from build123d import *

# Parameters (mm, degrees)
SKETCH1_W           = 604.52
SKETCH1_H           = 251.46
BOSS_EXTRUDE1_DEPTH = 35.56
SKETCH2_W           = 601.98
SKETCH2_H           = 248.92
CUT_EXTRUDE1_DEPTH  = 34.29
SKETCH3_W           = 101.6
SKETCH3_H           = 6.35
BOSS_EXTRUDE2_DEPTH = 30.48
SKETCH4_W           = 88.9
SKETCH4_H           = 21.59
CUT_EXTRUDE2_DEPTH  = 341.808114523
FILLET1_R           = 5.08
FILLET2_R           = 5.08


with BuildPart() as part:
    # Sketch1 → Boss-Extrude1 (new body)
    with BuildSketch(Plane(origin=(0, 0, 0), x_dir=(1, 0, 0), z_dir=(0, 1, 0))):
        Rectangle(SKETCH1_W, SKETCH1_H)
    extrude(amount=-BOSS_EXTRUDE1_DEPTH)

    # Sketch2 → Cut-Extrude1 (cut)
    with BuildSketch(Plane(origin=(0, 0, 0), x_dir=(1, 0, 0), z_dir=(0, 1, 0))):
        Rectangle(SKETCH2_W, SKETCH2_H)
    extrude(amount=-CUT_EXTRUDE1_DEPTH, mode=Mode.SUBTRACT)

    # Sketch3 → Boss-Extrude2 (add)
    with BuildSketch(Plane.XY.offset(125.73)):
        with Locations((-175.26, -19.05)):
            Rectangle(SKETCH3_W, SKETCH3_H)
        with Locations((175.26, -19.05)):
            Rectangle(SKETCH3_W, SKETCH3_H)
    extrude(amount=BOSS_EXTRUDE2_DEPTH)

    # Sketch4 → Cut-Extrude2 (cut, through all)
    with BuildSketch(Plane(origin=(0, -15.875, 0), x_dir=(1, 0, 0), z_dir=(0, 1, 0))):
        with Locations((-175.26, -139.065)):
            Rectangle(SKETCH4_W, SKETCH4_H)
        with Locations((175.26, -139.065)):
            Rectangle(SKETCH4_W, SKETCH4_H)
    extrude(amount=-CUT_EXTRUDE2_DEPTH, mode=Mode.SUBTRACT)

    # Fillet1
    fillet1_edges = [part.edges().sort_by_distance(p)[0] for p in [
        (-219.71, -19.05, 149.86),
        (-219.71, -19.05, 128.27),
        (-130.81, -19.05, 128.27),
        (-130.81, -19.05, 149.86),
        (219.71, -19.05, 128.27),
        (219.71, -19.05, 149.86),
        (130.81, -19.05, 149.86),
        (130.81, -19.05, 128.27),
    ]]
    fillet(fillet1_edges, radius=FILLET1_R)

    # Fillet2
    fillet2_edges = [part.edges().sort_by_distance(p)[0] for p in [
        (-226.06, -19.05, 156.21),
        (-124.46, -19.05, 156.21),
        (226.06, -19.05, 156.21),
        (124.46, -19.05, 156.21),
    ]]
    fillet(fillet2_edges, radius=FILLET2_R)


solid = part.part
Check sheet for the modelled part. Datum: model origin and axes. Units: mm. A direction names the side the tool comes from. Give positions to 0.01 mm unless a question says otherwise; leave off trailing zeros. Loops run counter-clockwise (first coordinate to the right, second up) from the corner with the lowest first, then second, coordinate; pieces in that order, holes last. Notation, with made-up numbers: M 64.25,29 L 102.25,29 A24 cw 102.25,50 Z; hole C 19,89.25 d1. An arc over 180 degrees is marked long. Return JSON: item names as keys, results as strings. Group by question number.
1. Go/stop test with flat-tipped pins: pin 1 (5 mm diameter, centred on x = 73.5, y = -30.5, fed in from +Z); pin 2 (7 mm diameter, centred on y = -19, z = 140, fed in from -X); pin 3 (7 mm diameter, centred on y = -18.5, z = 140, fed in from +X). Record where each tip stops, or that it passes through.
2. Cross-section at B-B on y = -7.5. Record the boundary of the cut face in (x, z), plus the area to 3 significant figures.
3. Mould release check, pull along X, two halves, no side actions. Record for faces 5 (the flat face through (-4, -18, -125.73)), 6 (the flat face through (-4, -17, -124.46)), 7 (the flat face through (302.26, -18, 2)): released by +X, released by -X, zero draft, split by the parting line, or undercut.
4. Tool access check on faces 1 (the flat face through (-176, -15.875, 151)), 2 (the flat face through (300.99, -17, 2)), 3 (the flat face through (-176, -22.225, 151)), 4 (the flat face through (-302.26, -18, 2)). Record the directions out of +Z, -Z, +X, -X, +Y, -Y that give a thin tool (end or side, any length) a straight path to the whole face; none if there is none.
5. Cross-section at D-D on z = -38. Record the boundary of the cut face in (x, y), plus the area to 3 significant figures.
6. Cross-section at C-C on x = 256.5. Record the boundary of the cut face in (y, z).
7. Cross-section at A-A on x = 150.5. Record the boundary of the cut face in (y, z) (3 decimals).
8. Thickness scan on L1, parallel to X at y = -24, z = -87; L2, parallel to Z at x = -65.5, y = -24.5; L3, parallel to Y at x = -21.5, z = 60. Record the ranges inside material, lowest first.
Return value:
{
 "1": {"pin 1": "z = 125.73", "pin 2": "x = -226.06", "pin 3": "x = 226.06"},
 "2": {"outline": "M -302.26,-125.73 L 302.26,-125.73 L 302.26,125.73 L -302.26,125.73 Z; hole M -300.99,-124.46 L 300.99,-124.46 L 300.99,124.46 L -300.99,124.46 Z", "area": "2,170 mm^2"},
 "3": {"face 5": "zero draft", "face 6": "undercut", "face 7": "released by +X"},
 "4": {"face 1": "+Z, +X, -X, +Y", "face 2": "+Y", "face 3": "+Z, +X, -X, -Y", "face 4": "+Z, -Z, -X, +Y, -Y"},
 "5": {"outline": "M -302.26,-35.56 L 302.26,-35.56 L 302.26,0 L 300.99,0 L 300.99,-34.29 L -300.99,-34.29 L -300.99,0 L -302.26,0 Z", "area": "855 mm^2"},
 "6": {"outline": "M -35.56,-125.73 L 0,-125.73 L 0,-124.46 L -34.29,-124.46 L -34.29,124.46 L 0,124.46 L 0,125.73 L -35.56,125.73 Z"},
 "7": {"outline": "M -35.56,-125.73 L 0,-125.73 L 0,-124.46 L -34.29,-124.46 L -34.29,124.46 L 0,124.46 L 0,125.73 L -15.875,125.73 L -15.875,128.27 L -22.225,128.27 L -22.225,125.73 L -35.56,125.73 Z; M -22.225,149.86 L -15.875,149.86 L -15.875,156.21 L -22.225,156.21 Z"},
 "8": {"L1": "-302.26 to -300.99, 300.99 to 302.26", "L2": "-125.73 to -124.46, 124.46 to 125.73", "L3": "-35.56 to -34.29"}
}
